Design review of the part built by this model. Coordinates are the model's own, in mm. A direction names the side the tool comes from. Coordinates: 2 decimals unless noted, no trailing zeros. Write each loop counter-clockwise with the first axis right and the second up, starting at its lowest first coordinate (ties: lowest second). Pieces come first, ordered by that corner, then holes. Notation, with made-up numbers: (82, 73.25) - (140, 73.25) arc R13 ccw to (140, 81.25) - close; hole circle Ø7 at (68.25, 63.25). An arc over 180 degrees is marked (long way). Answer as a JSON object with one key per item and string values.
```python
from build123d import *

# Parameters (mm, degrees)
RESSALTO_EXTRUS_O1_DEPTH = 40
ESBO_O4_W                = 171.630568717
ESBO_O4_H                = 20
CORTE_EXTRUS_O3_DEPTH    = 10
ESBO_O5_W                = 100
ESBO_O5_H                = 15
RESSALTO_EXTRUS_O2_DEPTH = 45
ESBO_O6_R                = 10
CORTE_EXTRUS_O6_DEPTH    = 132.657158163
FILETE8_R                = 25
FILETE7_R                = 25
ESBO_O9_W                = 50
ESBO_O9_H                = 45
CORTE_EXTRUS_O7_DEPTH    = 5
FILETE9_R                = 25


with BuildPart() as part:
    # Esboço1 → Ressalto-extrusão1 (new body)
    with BuildSketch(Plane.XY):
        Polygon((-53.29532416, 9.300830565), (76.70467584, 9.300830565), (76.70467584, 66.378323073), (-53.29532416, 89.300830565), align=None)
    extrude(amount=RESSALTO_EXTRUS_O1_DEPTH)

    # Esboço4 → Corte-extrusão3 (cut)
    with BuildSketch(Plane(origin=(13.664290772, 77.494043834, 0), x_dir=(0.9848077530122075, -0.17364817766693377, 0), z_dir=(0.1736481776669338, 0.9848077530122076, 0))):
        with Locations((8.431345703, -20)):
            Rectangle(ESBO_O4_W, ESBO_O4_H)
    extrude(amount=-CORTE_EXTRUS_O3_DEPTH, mode=Mode.SUBTRACT)

    # Esboço5 → Ressalto-extrusão2 (add)
    with BuildSketch(Plane.XY.offset(40)):
        with Locations((-3.29532416, 16.800830565)):
            Rectangle(ESBO_O5_W, ESBO_O5_H)
    extrude(amount=RESSALTO_EXTRUS_O2_DEPTH)

    # Esboço6 → Corte-extrusão6 (cut, through all)
    with BuildSketch(Plane(origin=(0, 24.300830565, 0), x_dir=(1, 0, 0), z_dir=(0, 1, 0))):
        with Locations(Location((-28.29532416, -60, 0), (0, 0, 270))):
            Circle(ESBO_O6_R)
        with Locations(Location((21.70467584, -60, 0), (0, 0, 270))):
            Circle(ESBO_O6_R)
    extrude(amount=-CORTE_EXTRUS_O6_DEPTH, mode=Mode.SUBTRACT)

    # Filete8
    filete8_edges = [part.edges().sort_by_distance(p)[0] for p in [
        (46.70467584, 16.800830565, 85),
    ]]
    fillet(filete8_edges, radius=FILETE8_R)

    # Filete7
    filete7_edges = [part.edges().sort_by_distance(p)[0] for p in [
        (-53.29532416, 16.800830565, 85),
    ]]
    fillet(filete7_edges, radius=FILETE7_R)

    # Esboço9 → Corte-extrusão7 (cut)
    with BuildSketch(Plane(origin=(0, 24.300830565, 0), x_dir=(1, 0, 0), z_dir=(0, 1, 0))):
        with Locations((-28.29532416, -62.5)):
            Rectangle(ESBO_O9_W, ESBO_O9_H)
    extrude(amount=-CORTE_EXTRUS_O7_DEPTH, mode=Mode.SUBTRACT)

    # Filete9
    filete9_edges = [part.edges().sort_by_distance(p)[0] for p in [
        (-3.29532416, 21.800830565, 85),
    ]]
    fillet(filete9_edges, radius=FILETE9_R - 0.0001)  # a hair under: the kernel refuses the full size


solid = part.part
```
(1) Tool access review of faces 4 (the face through (46.705, 17, 50)), 5 (the face through (11, 73, 30)), 6 (the face through (4.22, 21.77, 77.87)), 7 (the face through (10, 24.301, 62)): name each direction out of +Z, -Z, +X, -X, +Y, -Y from which nothing blocks a thin tool from reaching the whole face with its end or side.
Solved:
{"face 4": "+Z, +X, +Y, -Y", "face 5": "+X, +Y", "face 6": "+Z, -X, +Y", "face 7": "+Z, +X, -X, +Y"}
(2) Take a section at B-B, the plane z = 43. Write out the cut boundary in (x, y).
Solved:
{"outline": "(-53.3, 9.3) - (46.7, 9.3) - (46.7, 24.3) - (-3.3, 24.3) - (-3.3, 19.3) - (-53.3, 19.3) - close"}
(3) To check wall thickness, follow line 1 (Z direction, x = 70.5, y = 63.5); line 2 (Z direction, x = -19, y = 64.5); line 3 (Y direction, x = 46.5, z = 57.5). State the ranges of each line that lie inside material, in increasing order. Write a range as from..to.
Solved:
{"line 1": "z = 0..10, 30..40", "line 2": "z = 0..40", "line 3": "y = 9.3..24.3"}
(4) Take a section at D-D, the plane y = 35. Write out the cut boundary in (x, z), and give its area (3 significant figures).
Solved:
{"outline": "(-53.3, 0) - (76.7, 0) - (76.7, 40) - (-53.3, 40) - close", "area": "5,200 mm^2"}
(5) Take a section at C-C, the plane x = 42.5. Write out the cut boundary in (y, z).
Solved:
{"outline": "(9.3, 0) - (72.41, 0) - (72.41, 10) - (62.26, 10) - (62.26, 30) - (72.41, 30) - (72.41, 40) - (24.3, 40) - (24.3, 73.88) - (9.3, 73.88) - close"}
(6) The part is to be moulded in two halves that separate along Z. For faces 1 (the face through (11, 73, 10)), 2 (the face through (-45.78, 14.37, 77.87)), 3 (the face through (11, 41, 0)), say which applies: pulls with the +Z half, pulls with the -Z half, needs draft (parallel to the pull), parting line crosses it, or undercut.
Solved:
{"face 1": "undercut", "face 2": "pulls with the +Z half", "face 3": "pulls with the -Z half"}
(7) Take a section at A-A, the plane z = 55.5. Write out the cut boundary in (x, y), and give its area (3 significant figures).
Solved:
{"outline": "(-53.3, 9.3) - (-37.23, 9.3) - (-37.23, 19.3) - (-53.3, 19.3) - close; (-19.37, 9.3) - (12.77, 9.3) - (12.77, 24.3) - (-3.3, 24.3) - (-3.3, 19.3) - (-19.37, 19.3) - close; (30.63, 9.3) - (46.7, 9.3) - (46.7, 24.3) - (30.63, 24.3) - close", "area": "803 mm^2"}
(8) For pin 1 (5 mm diameter, centred on x = 15, y = 19, fed in from -Z); pin 2 (22.5 mm diameter, centred on x = 2.5, z = 65.5, fed in from +Y); pin 3 (8 mm diameter, centred on x = 6.5, y = 35.5, fed in from +Z); pin 4 (4 mm diameter, centred on y = 22, z = 52, fed in from -X), all flat-tipped, find the tip position at first contact; note any pin that passes through.
Solved:
{"pin 1": "stops at z = 0", "pin 2": "stops at y = 24.3", "pin 3": "stops at z = 40", "pin 4": "stops at x = -3.3"}
